The model under review builds one solid part; all positions refer to its coordinate system, in mm. Round coordinates to 2 decimals unless told otherwise and drop trailing zeros. Write each loop counter-clockwise with the first axis right and the second up, starting at its lowest first coordinate (ties: lowest second). Pieces come first, ordered by that corner, then holes. Notation, with made-up numbers: (52.5, 52) - (108.5, 52) arc R12 cw to (108.5, 66) - close; hole circle Ø4 at (62.25, 2). An arc over 180 degrees is marked (long way). Return JSON: item names as keys, results as strings.
Autodesk Inventor part; units mm, degrees
ref_plane "YZ Plane" through (0, 0, 0) normal (1, 0, 0) x (0, 1, 0)
ref_plane "XZ Plane" through (0, 0, 0) normal (0, 1, 0) x (-1, 0, 0)
ref_plane "XY Plane" through (0, 0, 0) normal (0, 0, 1) x (1, 0, 0)
sketch "Sketch1" plane through (0, 0, 0) normal (0, 1, 0) x (-1, 0, 0)
  line L0 (0, 0) -> (120, 0)
  line L1 (120, 0) -> (120, 27)
  line L2 (120, 27) -> (0, 27)
  line L3 (0, 27) -> (0, 0)
  dimension "d5" = 120
  dimension "d6" = 27
extrude "Extrusion1" add sketch "Sketch1" along normal blind 3
sketch "Sketch2" plane through (0, 0, 0) normal (0, -1, 0) x (1, 0, 0)
  line L0 (-120, 27) -> (0, 27)
  line L1 (0, 27) -> (-6, 27)
  line L2 (-6, 27) -> (-6, 21)
  line L3 (-6, 21) -> (0, 21)
  line L4 (0, 21) -> (0, 27)
  point P0 (0, 0)
  dimension "d7" = 6
  dimension "d8" = 6
extrude "Extrusion2" cut sketch "Sketch2" along normal through all both and the other way through all
sketch "Sketch3" plane through (0, 0, 0) normal (0, -1, 0) x (1, 0, 0)
  line L0 (0, 0) -> (-120, 0)
  line L1 (-108, 0) -> (-96, 0)
  line L2 (-96, 0) -> (-96, -6)
  line L3 (-96, -6) -> (-108, -6)
  line L4 (-108, -6) -> (-108, 0)
  line L5 (-12, 0) -> (-24, 0)
  line L6 (-24, 0) -> (-24, -6)
  line L7 (-24, -6) -> (-12, -6)
  line L8 (-12, -6) -> (-12, 0)
  line L9 (0, 21) -> (0, 0)
  line L10 (-120, 0) -> (-120, 27)
  dimension "d11" = 12
  dimension "d12" = 6
  dimension "d13" = 12
  dimension "d14" = 6
  dimension "d15" = 12
  dimension "d16" = 12
extrude "Extrusion3" add sketch "Sketch3" against normal blind 3
properties part number "ramp-support"
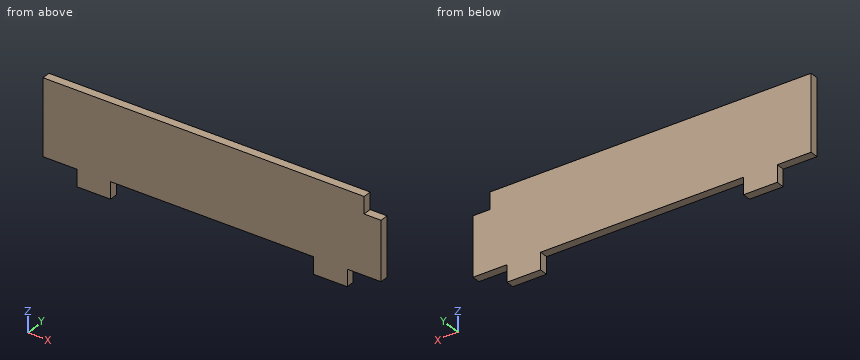
(1) Add section B-B (x = -82.5). Write out the cut boundary in (y, z).
Filled in:
{"outline": "(0, 0) - (3, 0) - (3, 27) - (0, 27) - close"}
(2) Wall thickness on line 1 (X direction, y = 2.35, z = -1); line 2 (Z direction, x = -28, y = 2.3); line 3 (X direction, y = 1.45, z = 25): over which ranges is each line inside the solid? List them lowest first.
Filled in:
{"line 1": "x = -108 to -96, -24 to -12", "line 2": "z = 0 to 27", "line 3": "x = -120 to -6"}
(3) Clearance check with flat-ended pins moving along their axes: pin 1 Ø1.5 at (x, y) = (-59.5, 1) entering from -Z; pin 2 Ø1.5 at (y, z) = (2, -3.5) entering from +X; pin 3 Ø0.9 at (y, z) = (2, -3) entering from -X; pin 4 Ø5 at (x, z) = (-103, 0.5) entering from -Y. State where each tip first meets the part, or that it passes through.
Filled in:
{"pin 1": "stops at z = 0", "pin 2": "stops at x = -12", "pin 3": "stops at x = -108", "pin 4": "stops at y = 0"}
(4) Add section A-A (y = 2.05). Write out the cut boundary in (x, z).
Filled in:
{"outline": "(-120, 0) - (-108, 0) - (-108, -6) - (-96, -6) - (-96, 0) - (-24, 0) - (-24, -6) - (-12, -6) - (-12, 0) - (0, 0) - (0, 21) - (-6, 21) - (-6, 27) - (-120, 27) - close"}
(5) Add section C-C (z = 23). Write out the cut boundary in (x, y), plus the area to 3 significant figures.
Filled in:
{"outline": "(-120, 0) - (-6, 0) - (-6, 3) - (-120, 3) - close", "area": "342 mm2"}
